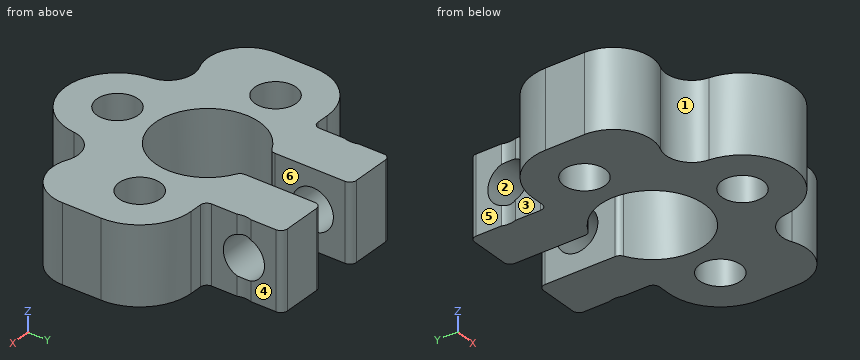
Autodesk Inventor part; units mm, degrees
ref_plane "YZ Plane" through (0, 0, 0) normal (1, 0, 0) x (0, 1, 0)
ref_plane "XZ Plane" through (0, 0, 0) normal (0, 1, 0) x (-1, 0, 0)
ref_plane "XY Plane" through (0, 0, 0) normal (0, 0, 1) x (1, 0, 0)
sketch "スケッチ1" plane through (0, 0, 0) normal (0, 0, 1) x (1, 0, 0)
  arc A0 (-1.55, 3.7417) -> (1.55, 3.7417) centre (0, 0) ccw
  circle A1 centre (-7, 0) radius 1.6
  circle A2 centre (7, 0) radius 1.6
  arc A3 (-7, 4) -> (-11, 0) centre (-7, 0) ccw
  arc A4 (11, 0) -> (7, 4) centre (7, 0) ccw
  line L0 (-1.55, 10) -> (-1.55, 3.7417)
  line L1 (1.55, 10) -> (1.55, 3.7417)
  circle A5 centre (0, -7) radius 1.6
  line L2 (1.55, 10) -> (5.55, 10)
  line L3 (5.55, 10) -> (5.55, 7.5385)
  line L4 (5.55, 4) -> (7, 4)
  line L5 (-1.55, 10) -> (-5.55, 10)
  line L6 (-5.55, 10) -> (-5.55, 7.5385)
  line L7 (-5.55, 4) -> (-7, 4)
  line L8 (-11, 0) -> (-11, -3)
  arc A6 (-11, -3) -> (-6.7837, -5.7424) centre (-8, -3) ccw
  arc A7 (1.55, 3.7417) -> (-1.55, 3.7417) centre (0, 0) ccw construction
  arc A8 (-3.9819, -7.3804) -> (3.9819, -7.3804) centre (0, -7) ccw
  arc A9 (-3.9819, -7.3804) -> (-6.7837, -5.7424) centre (-5.9728, -7.5706) ccw
  line L9 (11, 0) -> (11, -3)
  arc A10 (6.7837, -5.7424) -> (11, -3) centre (8, -3) ccw
  arc A11 (6.7837, -5.7424) -> (3.9819, -7.3804) centre (5.9728, -7.5706) ccw
  arc A12 (-5.55, 7.5385) -> (-5.55, 6.4615) centre (-6.95, 7) ccw construction
  arc A13 (5.55, 6.4615) -> (5.55, 7.5385) centre (6.95, 7) ccw construction
  arc A14 (-5.55, 6.4615) -> (-5.55, 7.5385) centre (-6.95, 7) ccw
  arc A15 (5.55, 7.5385) -> (5.55, 6.4615) centre (6.95, 7) ccw
  line L10 (5.55, 6.4615) -> (5.55, 4)
  line L11 (5.55, 7.5385) -> (5.55, 6.4615) construction
  line L12 (-5.55, 6.4615) -> (-5.55, 4)
  line L13 (-5.55, 7.5385) -> (-5.55, 6.4615) construction
  dimension "d0" = 8.1
  dimension "d1" = 3.2
  dimension "d2" = 3.2
  dimension "d4" = 7
  dimension "d5" = 7
  dimension "d6" = 3.2
  dimension "d7" = 7
  dimension "d8" = 6
  dimension "d9" = 4
  dimension "d10" = 3.1
  dimension "d11" = 4
  dimension "d12" = 4
  dimension "d13" = 1.55
  dimension "d14" = 3
  dimension "d15" = 3
  dimension "d16" = 4
  dimension "d17" = 4
  dimension "d18" = 3
  dimension "d19" = 3
  dimension "d20" = 2
  dimension "d21" = 2
  dimension "d22" = 3
  dimension "d23" = 3
  dimension "d24" = 1.4
  dimension "d25" = 1.4
  dimension "d26" = 3
  dimension "d27" = 3
extrude "押し出し1" add sketch "スケッチ1" along normal blind 6
sketch "スケッチ2" plane through (5.55, 4, 0) normal (1, 0, 0) x (0, 0, -1)
  circle A0 centre (-3, 3) radius 1.6
  line L0 (0, 6) -> (-6, 6)
  point P0 (0, -4)
  dimension "d30" = 3.2
  dimension "d31" = 3
  dimension "d32" = 3
extrude "押し出し2" cut sketch "スケッチ2" against normal through all
fillet "フィレット1" radius 0.5 8 edges at (-5.55, 10, 3) (-1.55, 10, 3) (1.55, 10, 3) (5.55, 10, 3) (5.55, 4, 3) (-5.55, 4, 3) (-1.55, 3.7417, 3) (1.55, 3.7417, 3)
properties part number "カップリング_軸8mm"
Source: CAD feature listing. Evaluate the final solid. Frame: model axes, mm. Face numbers are marked on the shaded views. A direction names the side the tool comes from. Coordinates: 2 decimals unless noted, no trailing zeros. Loops run counter-clockwise (first coordinate to the right, second up) from the corner with the lowest first, then second, coordinate; pieces in that order, holes last. Notation, with made-up numbers: (62.5, 74.25) -> (74.5, 74.25) arc R36 cw to (74.5, 111.25) -> close; hole circle Ø2 at (50.25, 71). An arc over 180 degrees is marked (long way). Answer in a Markdown table with one row per item. Add a question column.
Q1. Pull-direction query (Y, two-part tool) for the marked faces 1, 2 and 3; classes: pulls with the +Y half, pulls with the -Y half, needs draft (parallel to the pull), parting line crosses it, or undercut.
Q2. Section A-A on y = 7. Return the cut outline in (x, z).
Q3. Section B-B on x = 0. Return the cut outline in (y, z).
Q4. Section D-D on x = 3.5. Return the cut outline in (y, z).
Q5. Contact query for flat-ended pins moving along their axis: pin 1 Ø3 at (x, y) = (0, -7) entering from -Z; pin 2 Ø2 at (y, z) = (8.5, 3) entering from -X; pin 3 Ø0.5 at (x, z) = (6.5, 3) entering from +Y; pin 4 Ø3 at (y, z) = (-8, 4) entering from +X. Output: stop coordinate, or through.
Q6. Ray query, line 1 along Y through (x, z) = (0, 2.85); line 2 along Z through (x, y) = (-2.4, 7); line 3 along X through (y, z) = (-5.75, 2.25). Return the intervals inside material, ascending.
Q7. Section C-C on z = 5.75. Give the number of separate pieces and of enclosed holes in the cut face, and give its area (3 significant figures).
Q8. Reachability of the marked faces 4, 5 and 6 from +Z, -Z, +X, -X, +Y, -Y: full face, straight path, thin tool, end or side. Return the list, or none.
Computed values:
| question | item | result |
|---|---|---|
| 1 | face 1 | pulls with the -Y half |
| 1 | face 2 | undercut |
| 1 | face 3 | needs draft |
| 2 | outline | (-5.45, 0) -> (-1.55, 0) -> (-1.55, 1.4) -> (-5.45, 1.4) -> close; (-5.45, 4.6) -> (-1.55, 4.6) -> (-1.55, 6) -> (-5.45, 6) -> close; (1.55, 0) -> (5.45, 0) -> (5.45, 1.4) -> (1.55, 1.4) -> close; (1.55, 4.6) -> (5.45, 4.6) -> (5.45, 6) -> (1.55, 6) -> close |
| 3 | outline | (-11, 0) -> (-8.6, 0) -> (-8.6, 6) -> (-11, 6) -> close; (-5.4, 0) -> (-4.05, 0) -> (-4.05, 6) -> (-5.4, 6) -> close |
| 4 | outline | (-8.94, 0) -> (-2.04, 0) -> (-2.04, 6) -> (-8.94, 6) -> close; (2.04, 0) -> (10, 0) -> (10, 6) -> (2.04, 6) -> close; hole circle Ø3.2 at (7, 3) |
| 5 | pin 1 | passes through |
| 5 | pin 2 | stops at x = -5.55 |
| 5 | pin 3 | stops at y = 4 |
| 5 | pin 4 | stops at x = 4.28 |
| 6 | line 1 | y = -11 to -8.6, -5.4 to -4.05 |
| 6 | line 2 | z = 0 to 1.4, 4.6 to 6 |
| 6 | line 3 | x = -9.2 to -6.8, -5.14 to -1, 1 to 5.14, 6.8 to 9.2 |
| 7 | separate pieces | 1 |
| 7 | enclosed holes | 3 |
| 7 | area | 213 mm^2 |
| 8 | face 4 | +Z, -Z, +X, +Y |
| 8 | face 5 | +Z, -Z, -X, +Y |
| 8 | face 6 | +Z, -Z, +Y |
